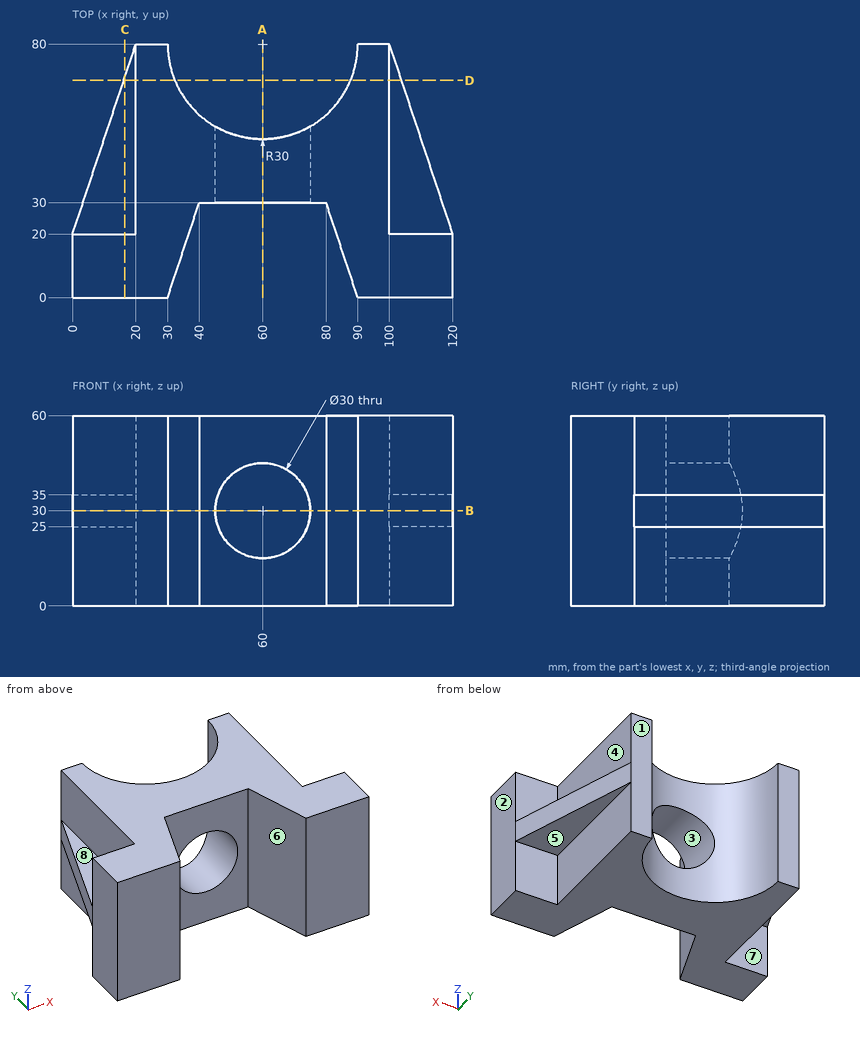
Geometry check sheet. Reference: drawing and pictorial views, mm from the part's lowest x, y, z. A direction names the side the tool comes from. Coordinates: 2 decimals unless noted, no trailing zeros. Order: outer loops, then holes, each group sorted by start corner. A loop starts at its lowest first (then second) coordinate and runs counter-clockwise, first axis right, second up.
1. Sectioned sample at C-C, the plane x = 16.5. Record the cut outline in (y, z), and give its area (4 significant figures).
Results found:
outline: (0, 0) - (20, 0) - (20, 25) - (69.5, 25) - (69.5, 35) - (20, 35) - (20, 60) - (0, 60) - close
area: 1,695 mm2
2. Scan lines: line 1 (Z direction, x = 60, y = 39); line 2 (Y direction, x = 11.5, z = 20.5); line 3 (X direction, y = 75.5, z = 14.5). Record each from-to range of solid material in increasing order.
Results found:
line 1: z = 0 to 15, 45 to 60
line 2: y = 0 to 20
line 3: x = 20 to 30.34, 89.66 to 100
3. Go/stop test with flat-tipped pins: pin 1 Ø10 at (x, y) = (13, 52) entering from -Z; pin 2 Ø6 at (x, y) = (109.5, 50) entering from +Z; pin 3 Ø22 at (x, y) = (11.5, 39) entering from -Z; pin 4 Ø2 at (y, z) = (49.5, 30) entering from -X. Record where each tip stops, or that it passes through.
Results found:
pin 1: stops at z = 25
pin 2: stops at z = 35
pin 3: stops at z = 0
pin 4: stops at x = 9.5
4. Release check for a two-part mould opening along X. For the marked faces 1, 2 and 3 record: +X half, -X half, draft (parallel to the pull), parting line (faces both ways), or undercut.
Results found:
face 1: draft
face 2: +X half
face 3: undercut
5. Set-up check for the marked faces 4, 5, 6, 7 and 8: record each of +Z, -Z, +X, -X, +Y, -Y from which the full face is reachable in a straight line by a thin tool's end or side.
Results found:
face 4: +Z, +X, +Y
face 5: -Z, +X, +Y
face 6: +Z, -Z, -Y
face 7: -Z, -X, +Y
face 8: +Z, -X, +Y
6. Sectioned sample at B-B, the plane z = 30. Record the cut outline in (x, y).
Results found:
outline: (0, 0) - (30, 0) - (40, 30) - (45, 30) - (45, 54.02) arc R30 cw to (30, 80) - (20, 80) - (0, 20) - close; (75, 30) - (80, 30) - (90, 0) - (120, 0) - (120, 20) - (100, 80) - (90, 80) arc R30 cw to (75, 54.02) - close
7. Sectioned sample at A-A, the plane x = 60. Record the cut outline in (y, z), and give its area (3 significant figures).
Results found:
outline: (30, 0) - (50, 0) - (50, 15) - (30, 15) - close; (30, 45) - (50, 45) - (50, 60) - (30, 60) - close
area: 600 mm2
8. Sectioned sample at D-D, the plane y = 68.5. Record the cut outline in (x, z), and give its area (3 significant figures).
Results found:
outline: (16.17, 25) - (20, 25) - (20, 0) - (32.29, 0) - (32.29, 60) - (20, 60) - (20, 35) - (16.17, 35) - close; (87.71, 0) - (100, 0) - (100, 25) - (103.83, 25) - (103.83, 35) - (100, 35) - (100, 60) - (87.71, 60) - close
area: 1,550 mm2
